The model under review builds one solid part; all positions refer to its coordinate system, in mm. Face numbers are marked on the shaded views. A direction names the side the tool comes from. Coordinates: 2 decimals unless noted, no trailing zeros. Loops run counter-clockwise (first coordinate to the right, second up) from the corner with the lowest first, then second, coordinate; pieces in that order, holes last. Notation, with made-up numbers: M 72,66.25 L 109,66.25 A22 ccw 109,73.25 Z; hole C -16,28 d10. An arc over 180 degrees is marked long. One line per item, written item: value.
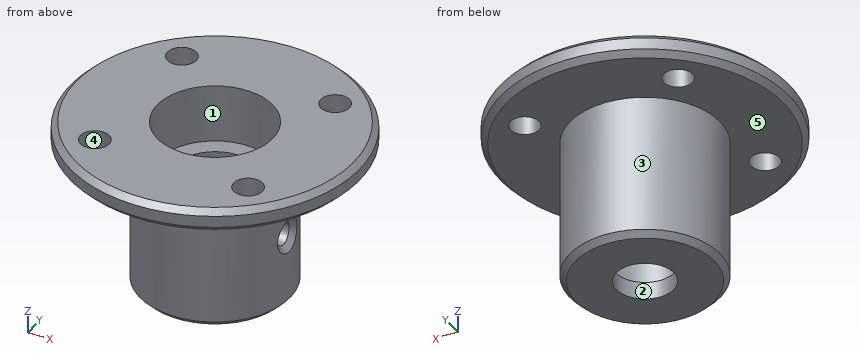
Autodesk Inventor part; units mm, degrees
ref_plane "YZ Plane" through (0, 0, 0) normal (1, 0, 0) x (0, 1, 0)
ref_plane "XZ Plane" through (0, 0, 0) normal (0, 1, 0) x (-1, 0, 0)
ref_plane "XY Plane" through (0, 0, 0) normal (0, 0, 1) x (1, 0, 0)
sketch "Sketch1" plane through (0, 0, 0) normal (0, 0, 1) x (1, 0, 0)
  circle A0 centre (0, 0) radius 12.5
  dimension "d0" = 25
extrude "Extrusion1" add sketch "Sketch1" along normal blind 2
sketch "Sketch2" plane through (0, 0, 0) normal (0, 0, -1) x (-1, 0, 0)
  circle A0 centre (0, 0) radius 12.5
  circle A1 centre (0, 0) radius 6.5
  dimension "d3" = 13
extrude "Extrusion2" add sketch "Sketch2" along normal blind 12.5 contours A1
sketch "Sketch3" plane through (0, 0, 2) normal (0, 0, 1) x (1, 0, 0)
  circle A0 centre (0, 0) radius 12.5
  circle A1 centre (0, 0) radius 5
  dimension "d6" = 10
extrude "Extrusion3" cut sketch "Sketch3" against normal blind 5 contours A1
sketch "Sketch4" plane through (0, 0, -3) normal (0, 0, 1) x (1, 0, 0)
  circle A0 centre (0, 0) radius 5
  circle A1 centre (0, 0) radius 3.5
  dimension "d9" = 7
extrude "Extrusion4" cut sketch "Sketch4" against normal blind 8 contours A1
sketch "Sketch5" plane through (0, 0, -11) normal (0, 0, 1) x (1, 0, 0)
  circle A0 centre (0, 0) radius 3.5
  circle A1 centre (0, 0) radius 2.5
  dimension "d12" = 5
extrude "Extrusion5" cut sketch "Sketch5" against normal through all contours A1
sketch "Sketch6" plane through (0, 0, 0) normal (1, 0, 0) x (0, 1, 0)
  line L0 (-6.5, -12.5) -> (6.5, -12.5)
  line L1 (6.5, 0) -> (-6.5, 0)
  line L2 (6.5, 0) -> (6.5, -12.5)
  line L3 (-6.5, 0) -> (-6.5, -12.5)
  point P0 (0, 0)
  point P1 (0, -6.25)
hole "Hole1" at (0, 0, -6.25) direction (1, 0, 0) diameter 2 end through all
chamfer "Chamfer1" distance 0.5 angle 45 4 edges at (-12.5, 0, 2) (-12.5, 0, 0) (6.5, 0, -12.5) (6.5, 0.0019, -7.25)
sketch "Sketch7" plane through (0, 0, 2) normal (0, 0, 1) x (1, 0, 0)
  circle A0 centre (0, 0) radius 12
  circle A1 centre (0, 0) radius 9.5
  circle A2 centre (0, 0) radius 3.5 construction
  line L0 (0, 0) -> (12, 0) construction
  circle A3 centre (0, 0) radius 2.5 construction
  line L1 (0, 0) -> (6.7175, 6.7175) construction
  circle A4 centre (6.7175, 6.7175) radius 1.25
  circle A5 centre (6.7175, -6.7175) radius 1.25
  circle A6 centre (-6.7175, -6.7175) radius 1.25
  circle A7 centre (-6.7175, 6.7175) radius 1.25
  point P0 (0, 9.5)
  point P1 (0, -9.5)
  point P2 (-9.5, 0)
  point P3 (9.5, 0)
  dimension "d25" = 19
  dimension "d26" = 45
  dimension "d29" = 360
  dimension "d31" = 2.5
  dimension "d32" = 2.5
  dimension "d33" = 2.5
  dimension "d34" = 2.5
extrude "Extrusion6" cut sketch "Sketch7" against normal through all contours A4 A1 | A1 A4 | A5 A1 | A1 A5 | A7 A1 | A1 A7 | A6 A1 | A1 A6
properties part number "22 - Valve Disc Hub" material "Steel AISI 1020 108 ANLD"
(1) Add section D-D on z = -1.5. State the section outline as (x, y) points, then the cut area to 3 significant figures.
Checks:
outline: C 0,0 d13; hole C 0,0 d10
area: 54.2 mm^2
(2) Add section B-B on z = -4. State the section outline as (x, y) points.
Checks:
outline: C 0,0 d13; hole C 0,0 d7
(3) Tool access review of the marked faces 1 and 2: name each direction out of +Z, -Z, +X, -X, +Y, -Y from which nothing blocks a thin tool from reaching the whole face with its end or side.
Checks:
face 1: +Z
face 2: +Z, -Z
(4) Draft analysis for pull direction X (two halves, no side actions). For the marked faces 3, 4 and 5, state which applies: pulls with the +X half, pulls with the -X half, needs draft (parallel to the pull), parting line crosses it, or undercut.
Checks:
face 3: parting line crosses it
face 4: undercut
face 5: needs draft
(5) Add section C-C on y = 0. State how many separate pieces and enclosed holes the cut face has, then the cut area to 3 significant figures.
Checks:
separate pieces: 3
enclosed holes: 0
area: 92.0 mm^2
(6) Insertion check: pin 1 Ø11 at (x, y) = (0, 0) entering from +Z; pin 2 Ø3 at (x, y) = (-6.72, -6.72) entering from -Z; pin 3 Ø3 at (x, z) = (-3, -3) entering from -Y; pin 4 Ø2 at (x, y) = (6.72, 6.72) entering from +Z. Each pin has a flat end and moves straight along its axis. Give the tip position at first contact, or say it passes through.
Checks:
pin 1: z = 2
pin 2: z = 0
pin 3: y = -6.32
pin 4: through
(7) To check wall thickness, follow L1, parallel to Y at x = 0, z = -8.75; L2, parallel to X at y = -6, z = 1.25; L3, parallel to Y at x = 0, z = -11.7. State the ranges of each line that lie inside material, in increasing order. Write a range as [from, to].
Checks:
L1: [-6.5, -3.5], [3.5, 6.5]
L2: [-10.97, -7.74], [-5.69, 5.69], [7.74, 10.97]
L3: [-6.5, -2.5], [2.5, 6.5]
(8) Add section A-A on x = 0. State the section outline as (y, z) points, then the cut area to 4 significant figures.
Checks:
outline: M -12.5,0.5 L -12,0 L -6.5,0 L -6.5,-12 L -6,-12.5 L -2.5,-12.5 L -2.5,-11 L -3.5,-11 L -3.5,-3 L -5,-3 L -5,2 L -12,2 L -12.5,1.5 Z; M 2.5,-12.5 L 6,-12.5 L 6.5,-12 L 6.5,0 L 12,0 L 12.5,0.5 L 12.5,1.5 L 12,2 L 5,2 L 5,-3 L 3.5,-3 L 3.5,-11 L 2.5,-11 Z
area: 98.25 mm^2
